Part print with two shaded views. Sizes in mm from the minimum x, y, z corner. Give positions to 0.01 mm unless a question says otherwise; leave off trailing zeros. Order: outer loops, then holes, each group sorted by start corner. A loop starts at its lowest first (then second) coordinate and runs counter-clockwise, first axis right, second up. Notation, with made-up numbers: M 21,54 L 58,54 A11 ccw 58,59 Z; hole C 51.5,79.25 d10. An arc over 180 degrees is marked long. Return JSON: item names as keys, results as strings. Group by question number.
1. Slice it at C-C on x = 5. List the corners of the cut face in (y, z), then the cut area to 3 significant figures.
2. Slice it at B-B on y = 55. List the corners of the cut face in (x, z), then the cut area to 3 significant figures.
3. Slice it at A-A on x = 55. List the corners of the cut face in (y, z).
4. Slice it at D-D on z = 2.15. List the corners of the cut face in (x, y), then the cut area to 3 significant figures.
5. Wall check: probe 1 along Y at (x, z) = (55, 0.4); probe 2 along Y at (x, z) = (5, 0.5); probe 3 along Y at (x, z) = (5, 2). Give the ranges that are in metal, low to high. Write a range as [from, to].
6. Pin check, flat tip, straight feed: pin 1 (6 mm diameter, centred on x = 55, y = 55, fed in from +Z). Stop position of the tip, or through.
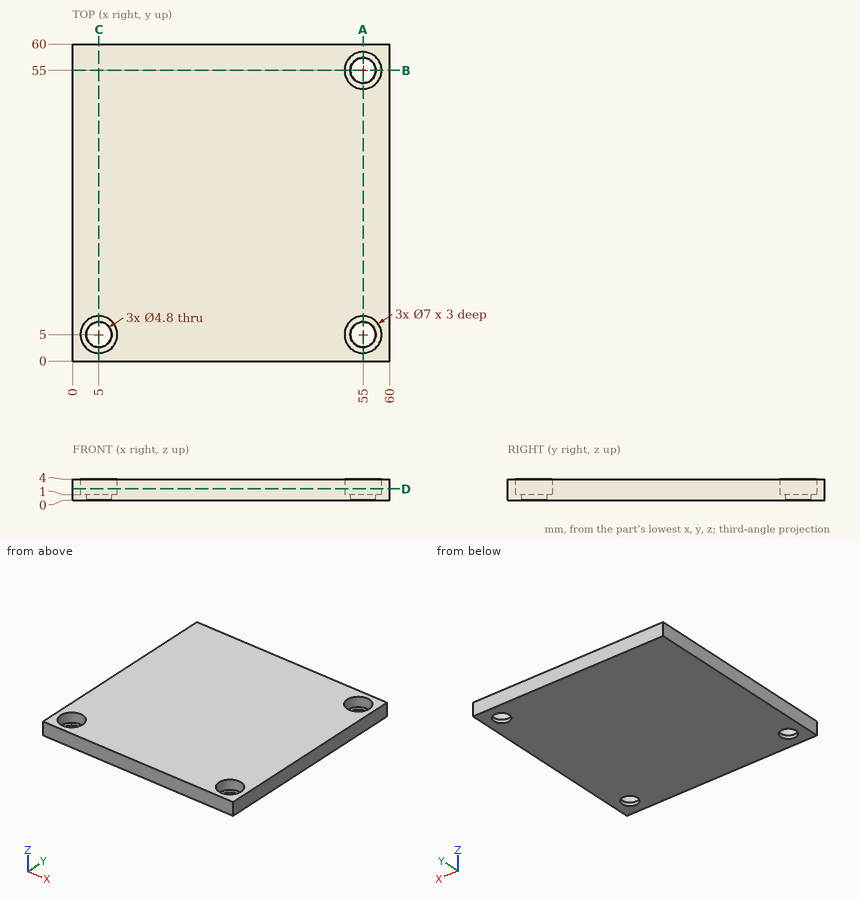
Result:
{
 "1": {"outline": "M 0,0 L 2.6,0 L 2.6,1 L 1.5,1 L 1.5,4 L 0,4 Z; M 7.4,0 L 60,0 L 60,4 L 8.5,4 L 8.5,1 L 7.4,1 Z", "area": "214 mm2"},
 "2": {"outline": "M 0,0 L 52.6,0 L 52.6,1 L 51.5,1 L 51.5,4 L 0,4 Z; M 57.4,0 L 60,0 L 60,4 L 58.5,4 L 58.5,1 L 57.4,1 Z", "area": "214 mm2"},
 "3": {"outline": "M 0,0 L 2.6,0 L 2.6,1 L 1.5,1 L 1.5,4 L 0,4 Z; M 7.4,0 L 52.6,0 L 52.6,1 L 51.5,1 L 51.5,4 L 8.5,4 L 8.5,1 L 7.4,1 Z; M 57.4,0 L 60,0 L 60,4 L 58.5,4 L 58.5,1 L 57.4,1 Z"},
 "4": {"outline": "M 0,0 L 60,0 L 60,60 L 0,60 Z; hole C 5,5 d7; hole C 55,5 d7; hole C 55,55 d7", "area": "3,480 mm2"},
 "5": {"probe 1": "y = [0, 2.6], [7.4, 52.6], [57.4, 60]", "probe 2": "y = [0, 2.6], [7.4, 60]", "probe 3": "y = [0, 1.5], [8.5, 60]"},
 "6": {"pin 1": "stops at z = 1"}
}
